Input: part model. Units: mm. Frame: model coordinates. A direction names the side the tool comes from. Give positions to 0.01 mm unless a question says otherwise; leave off trailing zeros. Write each loop counter-clockwise with the first axis right and the second up, starting at its lowest first coordinate (ties: lowest second). Pieces come first, ordered by that corner, then holes.
```python
from build123d import *

# Parameters (mm, degrees)
SKETCH_R        = 1.375
PAD_DEPTH       = 4
PAD001_DEPTH    = 12
SKETCH002_R     = 1.4
POCKET_DEPTH    = 8
SKETCH003_R     = 1.4
POCKET001_DEPTH = 8
FILLET_R        = 2
SKETCH004_R     = 3
POCKET002_DEPTH = 1.5
SKETCH005_R     = 1.4
POCKET003_DEPTH = 5
PAD002_DEPTH    = 16
SKETCH007_R     = 1.4
POCKET004_DEPTH = 8


with BuildPart() as part:
    # Sketch → Pad (new body)
    with BuildSketch(Plane.XY):
        with BuildLine():
            Line((-106, 65), (106, 65))
            ThreePointArc((110, 61), (108.828427, 63.828427), (106, 65))
            Line((110, 61), (110, -61))
            ThreePointArc((106, -65), (108.828427, -63.828427), (110, -61))
            Line((106, -65), (-106, -65))
            ThreePointArc((-110, -61), (-108.828427, -63.828427), (-106, -65))
            Line((-110, -61), (-110, 61))
            ThreePointArc((-106, 65), (-108.828427, 63.828427), (-110, 61))
        make_face()
        with Locations((-100, 60)):
            Circle(SKETCH_R, mode=Mode.SUBTRACT)
        with Locations((-28, 60)):
            Circle(SKETCH_R, mode=Mode.SUBTRACT)
        with Locations((67, 60)):
            Circle(SKETCH_R, mode=Mode.SUBTRACT)
        with Locations((67, 18)):
            Circle(SKETCH_R, mode=Mode.SUBTRACT)
        with Locations((-36, 18)):
            Circle(SKETCH_R, mode=Mode.SUBTRACT)
        with Locations((-100, 18)):
            Circle(SKETCH_R, mode=Mode.SUBTRACT)
        with BuildLine():
            ThreePointArc((-97, -7), (-99.828427, -8.171573), (-101, -11))
            Line((-101, -53), (-101, -11))
            ThreePointArc((-101, -53), (-99.828427, -55.828427), (-97, -57))
            Line((97, -57), (-97, -57))
            ThreePointArc((97, -57), (99.828427, -55.828427), (101, -53))
            Line((101, -11), (101, -53))
            ThreePointArc((101, -11), (99.828427, -8.171573), (97, -7))
            Line((-97, -7), (97, -7))
        make_face(mode=Mode.SUBTRACT)
        with BuildLine():
            ThreePointArc((-91, 55), (-93.828427, 53.828427), (-95, 51))
            Line((-95, 27), (-95, 51))
            ThreePointArc((-95, 27), (-93.828427, 24.171573), (-91, 23))
            Line((97, 23), (-91, 23))
            ThreePointArc((97, 23), (99.828427, 24.171573), (101, 27))
            Line((101, 51), (101, 27))
            ThreePointArc((101, 51), (99.828427, 53.828427), (97, 55))
            Line((-91, 55), (97, 55))
        make_face(mode=Mode.SUBTRACT)
    extrude(amount=PAD_DEPTH)

    # Sketch001 (on Face32 of Pad) → Pad001 (join)
    with BuildSketch(Plane.XY.offset(4)):
        with BuildLine():
            ThreePointArc((-109, 54.5), (-109.707107, 54.207107), (-110, 53.5))
            Line((-110, 41.5), (-110, 53.5))
            ThreePointArc((-110, 41.5), (-109.707107, 40.792893), (-109, 40.5))
            Line((-105, 40.5), (-109, 40.5))
            ThreePointArc((-105, 40.5), (-104.292893, 40.792893), (-104, 41.5))
            Line((-104, 53.5), (-104, 41.5))
            ThreePointArc((-104, 53.5), (-104.292893, 54.207107), (-105, 54.5))
            Line((-109, 54.5), (-105, 54.5))
        make_face()
        with BuildLine():
            ThreePointArc((-109, -40.5), (-109.707107, -40.792893), (-110, -41.5))
            Line((-110, -53.5), (-110, -41.5))
            ThreePointArc((-110, -53.5), (-109.707107, -54.207107), (-109, -54.5))
            Line((-105, -54.5), (-109, -54.5))
            ThreePointArc((-105, -54.5), (-104.292893, -54.207107), (-104, -53.5))
            Line((-104, -41.5), (-104, -53.5))
            ThreePointArc((-104, -41.5), (-104.292893, -40.792893), (-105, -40.5))
            Line((-109, -40.5), (-105, -40.5))
        make_face()
        with BuildLine():
            ThreePointArc((105, 5), (104.292893, 4.707107), (104, 4))
            Line((104, -64), (104, 4))
            ThreePointArc((104, -64), (104.292893, -64.707107), (105, -65))
            Line((106, -65), (105, -65))
            ThreePointArc((106, -65), (108.828427, -63.828427), (110, -61))
            Line((110, 4), (110, -61))
            ThreePointArc((110, 4), (109.707107, 4.707107), (109, 5))
            Line((105, 5), (109, 5))
        make_face()
    extrude(amount=PAD001_DEPTH)

    # Sketch002 (on Face7 of Pad001) → Pocket (cut)
    with BuildSketch(Plane(origin=(-110, 0, 0), x_dir=(0, -1, 0), z_dir=(-1, 0, 0))):
        with Locations((-47.5, 9)):
            Circle(SKETCH002_R)
        with Locations((47.5, 9)):
            Circle(SKETCH002_R)
    extrude(amount=-POCKET_DEPTH, mode=Mode.SUBTRACT)

    # Sketch003 (on Face59 of Pocket) → Pocket001 (cut)
    with BuildSketch(Plane.YZ.offset(110)):
        with Locations((-56, 10)):
            Circle(SKETCH003_R)
        with Locations((-4, 10)):
            Circle(SKETCH003_R)
    extrude(amount=-POCKET001_DEPTH, mode=Mode.SUBTRACT)

    # Fillet
    fillet_edges = [part.edges().sort_by_distance(p)[0] for p in [
        (110, 0, 0),
    ]]
    fillet(fillet_edges, radius=FILLET_R)

    # Sketch004 (on Face10 of Fillet) → Pocket002 (cut)
    with BuildSketch(Plane(origin=(0, 0, 0), x_dir=(1, 0, 0), z_dir=(0, 0, -1))):
        with Locations((-50, 0)):
            Circle(SKETCH004_R)
        with Locations((50, 0)):
            Circle(SKETCH004_R)
    extrude(amount=-POCKET002_DEPTH, mode=Mode.SUBTRACT)

    # Sketch005 (on Face10 of Pocket002) → Pocket003 (cut)
    with BuildSketch(Plane(origin=(0, 0, 0), x_dir=(1, 0, 0), z_dir=(0, 0, -1))):
        with Locations((-50, 0)):
            Circle(SKETCH005_R)
        with Locations((50, 0)):
            Circle(SKETCH005_R)
    extrude(amount=-POCKET003_DEPTH, mode=Mode.SUBTRACT)

    # Sketch006 (on Face4 of Pocket003) → Pad002 (join)
    with BuildSketch(Plane.XY.offset(4)):
        with BuildLine():
            ThreePointArc((109, 14), (109.707107, 14.292893), (110, 15))
            Line((110, 19), (110, 15))
            ThreePointArc((110, 19), (109.707107, 19.707107), (109, 20))
            Line((91, 20), (109, 20))
            ThreePointArc((91, 20), (90.292893, 19.707107), (90, 19))
            Line((90, 15), (90, 19))
            ThreePointArc((90, 15), (90.292893, 14.292893), (91, 14))
            Line((109, 14), (91, 14))
        make_face()
    extrude(amount=PAD002_DEPTH)

    # Sketch007 (on Face30 of Pad002) → Pocket004 (cut)
    with BuildSketch(Plane(origin=(0, 20, 0), x_dir=(-1, 0, 0), z_dir=(0, 1, 0))):
        with Locations((-98, 17)):
            Circle(SKETCH007_R)
    extrude(amount=-POCKET004_DEPTH, mode=Mode.SUBTRACT)


solid = part.part
```
Q1. Access query for faces 4 (the flat face through (104, -30, 10)), 5 (the flat face through (107, 5, 10)), 6 (the cylindrical face through (99.797, -55.859, 1.972)). Directions: +Z, -Z, +X, -X, +Y, -Y. A direction counts if a zero-diameter tool reaches every point of the face in a straight line with its end or side. Return the directions, or none.
Q2. Section A-A, the plane x = -84.5. Return the cut outline in (y, z), then the cut area to 3 significant figures.
Q3. Section D-D, the plane y = -44. Return the cut outline in (x, z).
Q4. Mould query, pull axis Y, two halves, no side actions, for faces 1 (the cylindrical face through (-93.859, 24.203, 1.972)), 2 (the flat face through (107, -30, 16)), 3 (the cylindrical face through (-108.859, -63.797, 2.986)). Classes: +Y half, -Y half, draft (parallel to the pull), parting line (faces both ways), or undercut.
Q5. Pin query (flat end, axial travel): pin 1 (2 mm diameter, centred on x = 107, z = 11.5, fed in from +Y); pin 2 (5 mm diameter, centred on x = -106, y = 49.5, fed in from +Z); pin 3 (2.5 mm diameter, centred on y = -47.5, z = 9, fed in from -X); pin 4 (1.6 mm diameter, centred on x = -28, y = 60, fed in from -Z). Return the tip coordinate at first contact, or that it passes through.
Q6. Section B-B, the plane y = 33. Return the cut outline in (x, z).
Q7. Material intervals for line 1 along Y through (x, z) = (-36, 1.6) (3 decimals); line 2 along Y through (x, z) = (-50, 2.7); line 3 along Y through (x, z) = (58, 2.5), sorted ascending.
Q8. Section C-C, the plane y = -25. Return the cut outline in (x, z).
Solutions:
1. face 4: +Z, -Y
1. face 5: +Z, +X, -X
1. face 6: +Z, -Z
2. outline: (-65, 2) arc R2 ccw to (-63, 0) - (-57, 0) - (-57, 4) - (-65, 4) - close; (-7, 0) - (23, 0) - (23, 4) - (-7, 4) - close; (55, 0) - (63, 0) arc R2 ccw to (65, 2) - (65, 4) - (55, 4) - close
2. area: 190 mm2
3. outline: (-110, 2) arc R2 ccw to (-108, 0) - (-101, 0) - (-101, 4) - (-104, 4) - (-104, 16) - (-110, 16) - close; (101, 0) - (108, 0) arc R2 ccw to (110, 2) - (110, 16) - (104, 16) - (104, 4) - (101, 4) - close
4. face 1: undercut
4. face 2: draft
4. face 3: -Y half
5. pin 1: stops at y = 20
5. pin 2: stops at z = 16
5. pin 3: stops at x = 104
5. pin 4: passes through
6. outline: (-110, 2) arc R2 ccw to (-108, 0) - (-95, 0) - (-95, 4) - (-110, 4) - close; (101, 0) - (108, 0) arc R2 ccw to (110, 2) - (110, 4) - (101, 4) - close
7. line 1: y = -64.96 to -57, -7 to 16.625, 19.375 to 23, 55 to 64.96
7. line 2: y = -65 to -57, -7 to -1.4, 1.4 to 23, 55 to 65
7. line 3: y = -65 to -57, -7 to 23, 55 to 65
8. outline: (-110, 2) arc R2 ccw to (-108, 0) - (-101, 0) - (-101, 4) - (-110, 4) - close; (101, 0) - (108, 0) arc R2 ccw to (110, 2) - (110, 16) - (104, 16) - (104, 4) - (101, 4) - close
